```python
from build123d import *

# Parameters (mm, degrees)
BOSS_EXTRUDE1_DEPTH = 1
SKETCH2_W           = 11
SKETCH2_H           = 49
CUT_EXTRUDE1_DEPTH  = 38.434743221
FILLET1_R           = 1.5
SKETCH3_R           = 1.6
CUT_EXTRUDE2_DEPTH  = 38.434743221


with BuildPart() as part:
    # Sketch1 → Boss-Extrude1 (new body)
    with BuildSketch(Plane(origin=(0, 0, 0), x_dir=(1, 0, 0), z_dir=(0, 1, 0))):
        Polygon((19.4, 0), (16.2, 18), (11, 27), (4.6, 32), (-4.6, 32), (-11, 27), (-16.2, 18), (-19.4, 0), (-16.2, -18), (-11, -27), (-4.6, -32), (4.6, -32), (11, -27), (16.2, -18), align=None)
    extrude(amount=BOSS_EXTRUDE1_DEPTH)

    # Sketch2 → Cut-Extrude1 (cut, through all)
    with BuildSketch(Plane(origin=(0, 1, 0), x_dir=(1, 0, 0), z_dir=(0, 1, 0))):
        Rectangle(SKETCH2_W, SKETCH2_H)
    extrude(amount=-CUT_EXTRUDE1_DEPTH, mode=Mode.SUBTRACT)

    # Fillet1
    fillet1_edges = [part.edges().sort_by_distance(p)[0] for p in [
        (5.5, 0.5, -24.5),
        (5.5, 0.5, 24.5),
        (-5.5, 0.5, 24.5),
        (-5.5, 0.5, -24.5),
    ]]
    fillet(fillet1_edges, radius=FILLET1_R)

    # Sketch3 → Cut-Extrude2 (cut, through all)
    with BuildSketch(Plane(origin=(0, 1, 0), x_dir=(1, 0, 0), z_dir=(0, 1, 0))):
        with Locations(Location((-11, 18, 0), (0, 0, 270))):
            Circle(SKETCH3_R)
        with Locations(Location((11, 18, 0), (0, 0, 90))):
            Circle(SKETCH3_R)
        with Locations(Location((-11, -18, 0), (0, 0, 90))):
            Circle(SKETCH3_R)
        with Locations(Location((11, -18, 0), (0, 0, 270))):
            Circle(SKETCH3_R)
    extrude(amount=-CUT_EXTRUDE2_DEPTH, mode=Mode.SUBTRACT)


solid = part.part
```
The listing builds one solid part. Answer for the finished solid, in the listing's coordinates (mm). A direction names the side the tool comes from. Give positions to 0.01 mm unless a question says otherwise; leave off trailing zeros. Order: outer loops, then holes, each group sorted by start corner. A loop starts at its lowest first (then second) coordinate and runs counter-clockwise, first axis right, second up.
1) Find section A-A on z = -4.5. Write down the section's boundary in (x, y), then the cut area to 3 significant figures.
Reported:
outline: (-18.6, 0) - (-5.5, 0) - (-5.5, 1) - (-18.6, 1) - close; (5.5, 0) - (18.6, 0) - (18.6, 1) - (5.5, 1) - close
area: 26.2 mm2
2) Find section D-D on x = -10. Write down the section's boundary in (y, z).
Reported:
outline: (0, -27.78) - (1, -27.78) - (1, -19.25) - (0, -19.25) - close; (0, -16.75) - (1, -16.75) - (1, 16.75) - (0, 16.75) - close; (0, 19.25) - (1, 19.25) - (1, 27.78) - (0, 27.78) - close
3) Consider line 1 along X through (y, z) = (0.4, 18); line 2 along Z through (x, y) = (4, 0.35); line 3 along Z through (x, y) = (-10, 0.45). Determine where each line is inside the solid, lowest interval first.
Reported:
line 1: x = -16.2 to -12.6, -9.4 to -5.5, 5.5 to 9.4, 12.6 to 16.2
line 2: z = -32 to -24.5, 24.5 to 32
line 3: z = -27.78 to -19.25, -16.75 to 16.75, 19.25 to 27.78
4) Determine the mould class of faces 3 (the face through (13.636, 0.493, -22.437)), 4 (the face through (-5.05, 0.49, -24.07)), 5 (the face through (-7.8, 0.5, 29.5)) for opening direction Z: pulls with the +Z half, pulls with the -Z half, needs draft (parallel to the pull), parting line crosses it, or undercut.
Reported:
face 3: pulls with the -Z half
face 4: undercut
face 5: pulls with the +Z half
5) Given P1, Ø1.9, axis at x = -11, z = -18, coming from the -Y side, flat-ended and moving along its own axis, determine where the tip first touches the part or whether it passes through.
Reported:
P1: passes through
6) Find section C-C on y = 0.25. Write down the section's boundary in (x, z), then the cut area to 3 significant figures.
Reported:
outline: (-19.4, 0) - (-16.2, -18) - (-11, -27) - (-4.6, -32) - (4.6, -32) - (11, -27) - (16.2, -18) - (19.4, 0) - (16.2, 18) - (11, 27) - (4.6, 32) - (-4.6, 32) - (-11, 27) - (-16.2, 18) - close; hole circle Ø3.2 at (-11, -18); hole circle Ø3.2 at (-11, 18); hole (-5.5, -23) arc R1.5 ccw to (-4, -24.5) - (4, -24.5) arc R1.5 ccw to (5.5, -23) - (5.5, 23) arc R1.5 ccw to (4, 24.5) - (-4, 24.5) arc R1.5 ccw to (-5.5, 23) - close; hole circle Ø3.2 at (11, -18); hole circle Ø3.2 at (11, 18)
area: 1,360 mm2
7) Find section B-B on x = -1.5. Write down the section's boundary in (y, z), then the cut area to 3 significant figures.
Reported:
outline: (0, -32) - (1, -32) - (1, -24.5) - (0, -24.5) - close; (0, 24.5) - (1, 24.5) - (1, 32) - (0, 32) - close
area: 15.0 mm2
8) For faces 1 (the face through (5.05, 0.49, 24.07)), 2 (the face through (17.778, 0.493, 9.126)), determine the directions among +Z, -Z, +X, -X, +Y, -Y from which every point of the face is accessible in a straight line to the end or side of a thin tool.
Reported:
face 1: +Y, -Y
face 2: +Z, +X, +Y, -Y
